```python
from build123d import *

# Parameters (mm, degrees)
SKETCH_7_R          = 5
EXTRUDE_5_DEPTH     = 20
SKETCH_8_W          = 60
SKETCH_8_H          = 40
EXTRUDE_7_DEPTH     = 5
SKETCH_9_W          = 5
SKETCH_9_H          = 40
EXTRUDE_8_DEPTH     = 300
SKETCH_10_W         = 60
SKETCH_10_H         = 40
EXTRUDE_9_DEPTH     = 5
SKETCH_11_R         = 5
EXTRUDE_10_DEPTH    = 20
SKETCH_12_R         = 5
CUT_EXTRUDE_1_DEPTH = 96


with BuildPart() as part:
    # Эскиз7 → Бобышка-Вытянуть5 (new body)
    with BuildSketch(Plane.XY):
        with Locations(Location((0, 0, 0), (0, 0, 180))):
            Circle(SKETCH_7_R)
    extrude(amount=EXTRUDE_5_DEPTH)

    # Эскиз8 → Бобышка-Вытянуть7 (add)
    with BuildSketch(Plane.XY.offset(20)):
        Rectangle(SKETCH_8_W, SKETCH_8_H)
    extrude(amount=EXTRUDE_7_DEPTH)

    # Эскиз9 → Бобышка-Вытянуть8 (add)
    with BuildSketch(Plane.XY.offset(25)):
        with Locations((-27.5, 0)):
            Rectangle(SKETCH_9_W, SKETCH_9_H)
        with Locations((27.5, 0)):
            Rectangle(SKETCH_9_W, SKETCH_9_H)
    extrude(amount=EXTRUDE_8_DEPTH)

    # Эскиз10 → Бобышка-Вытянуть9 (add)
    with BuildSketch(Plane.XY.offset(325)):
        Rectangle(SKETCH_10_W, SKETCH_10_H)
    extrude(amount=EXTRUDE_9_DEPTH)

    # Эскиз11 → Бобышка-Вытянуть10 (add)
    with BuildSketch(Plane.XY.offset(330)):
        with Locations(Location((0, 0, 0), (0, 0, 180))):
            Circle(SKETCH_11_R)
    extrude(amount=EXTRUDE_10_DEPTH)

    # Эскиз12 → Вырез-Вытянуть1 (cut)
    with BuildSketch(Plane(origin=(30, 0, 0), x_dir=(0, 0, -1), z_dir=(1, 0, 0))):
        with Locations((-90, 0)):
            Circle(SKETCH_12_R)
        with Locations(Location((-260, 0, 0), (0, 0, 90))):
            Circle(SKETCH_12_R)
    extrude(amount=-CUT_EXTRUDE_1_DEPTH, mode=Mode.SUBTRACT)


solid = part.part
```
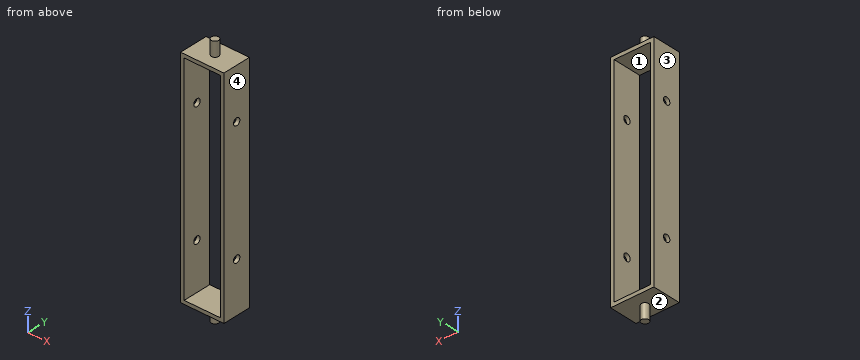
Here's how the part is built. I have some questions about the finished solid (model axes, mm). Face numbers are marked on the shaded views. Give positions to 0.01 mm unless a question says otherwise; leave off trailing zeros. Write each loop counter-clockwise with the first axis right and the second up, starting at its lowest first coordinate (ties: lowest second). Pieces come first, ordered by that corner, then holes. Notation, with made-up numbers: M 66,43 L 114,43 A26 cw 114,77 Z; hole C 31,86.5 d5. An arc over 180 degrees is marked long. Put each result on its own line as item: value. Start each with the question number.
Item 1: If we section it at C-C, the plane y = 0: Count the separate pieces of the cut face and the enclosed holes in it, then the cut area to 3 significant figures.
Item 2: If we section it at A-A, the plane x = 0: Write out the boundary of the cut face in (y, z).
Item 3: If we section it at B-B, the plane z = 260: Write out the boundary of the cut face in (x, y).
Item 4: Will these pins go through, and if not, where does the flat tip stop? pin 1 (6 mm diameter, centred on y = 0, z = 90, fed in from +X); pin 2 (4 mm diameter, centred on x = -15.5, y = -8, fed in from +Z).
Item 5: Thinking about a two-plate mould opening in X: for the marked faces 1, 2, 3 and 4, which applies, +X half, -X half, draft (parallel to the pull), parting line (faces both ways), or undercut?
Item 6: If we section it at D-D, the plane y = -14.5: Write out the boundary of the cut face in (x, z), then the cut area to 3 significant figures.
Item 7: I need wall thicknesses on L1, parallel to Z at x = 9, y = 3.5; L2, parallel to X at y = 1, z = 222; L3, parallel to Y at x = 28, z = 90. Which ranges of each line are inside material? Lowest first, please. Write a range as from..to.
Values:
1. separate pieces: 4
1. enclosed holes: 0
1. area: 3,800 mm²
2. outline: M -20,20 L -5,20 L -5,0 L 5,0 L 5,20 L 20,20 L 20,25 L -20,25 Z; M -20,325 L 20,325 L 20,330 L 5,330 L 5,350 L -5,350 L -5,330 L -20,330 Z
3. outline: M -30,-20 L -25,-20 L -25,-5 L -30,-5 Z; M -30,5 L -25,5 L -25,20 L -30,20 Z; M 25,-20 L 30,-20 L 30,-5 L 25,-5 Z; M 25,5 L 30,5 L 30,20 L 25,20 Z
4. pin 1: through
4. pin 2: z = 330
5. face 1: undercut
5. face 2: draft
5. face 3: -X half
5. face 4: +X half
6. outline: M -30,20 L 30,20 L 30,330 L -30,330 Z; hole M -25,25 L 25,25 L 25,325 L -25,325 Z
6. area: 3,600 mm²
7. L1: 20..25, 325..330
7. L2: -30..-25, 25..30
7. L3: -20..-5, 5..20
